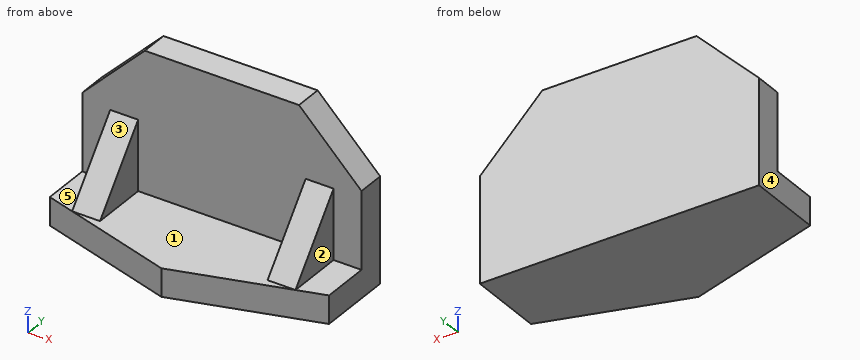
```python
from build123d import *

# Parameters (mm, degrees)
F0_W      = 127
F0_H      = 76.2
F1_DEPTH  = 53.848
F2_W      = 41.148
F2_H      = 63.5
F3_DEPTH  = 127
F5_DEPTH  = 12.7
F7_DEPTH  = 12.7
F8_W      = 12.7
F8_H      = 25.908
F9_DEPTH  = 31.75
F11_DEPTH = 12.7
F13_DEPTH = 12.7


with BuildPart() as f1:
    # F0 (on Front) → F1 (new body)
    with BuildSketch(Plane.XZ):
        with Locations((-17.504597, -0.584449)):
            Rectangle(F0_W, F0_H)
    extrude(amount=F1_DEPTH)

    # F2 (on face) → F3 (cut)
    with BuildSketch(Plane.YZ.offset(45.995403)):
        with Locations((-33.274, 5.765551)):
            Rectangle(F2_W, F2_H)
    extrude(amount=-F3_DEPTH, mode=Mode.SUBTRACT)

    # F4 (on face) → F5 (cut)
    with BuildSketch(Plane.XZ.offset(12.7)):
        Polygon((45.995403, 9.067551), (45.995403, 37.515551), (17.547403, 37.515551), align=None)
        Polygon((-52.556597, 37.515551), (-81.004597, 37.515551), (-81.004597, 9.067551), align=None)
    extrude(amount=-F5_DEPTH, mode=Mode.SUBTRACT)

    # F6 (on face) → F7 (cut)
    with BuildSketch(Plane.XY.offset(-25.984449)):
        Polygon((45.995403, -34.798), (-17.504597, -53.848), (45.995403, -53.848), align=None)
        Polygon((-81.004597, -53.848), (-17.504597, -53.848), (-81.004597, -34.798), align=None)
    extrude(amount=-F7_DEPTH, mode=Mode.SUBTRACT)

    # F8 (on face) → F9 (join)
    with BuildSketch(Plane.XY.offset(-25.984449)):
        with Locations((26.945403, -25.654)):
            Rectangle(F8_W, F8_H)
        with Locations((-61.954597, -25.654)):
            Rectangle(F8_W, F8_H)
    extrude(amount=F9_DEPTH)

    # F10 (on face) → F11 (cut)
    with BuildSketch(Plane.YZ.offset(-55.604597)):
        Polygon((-38.608, -25.984449), (-12.7, 5.765551), (-38.608, 5.765551), align=None)
    extrude(amount=-F11_DEPTH, mode=Mode.SUBTRACT)

    # F12 (on face) → F13 (cut)
    with BuildSketch(Plane.YZ.offset(33.295403)):
        Polygon((-38.608, -25.984449), (-12.7, 5.765551), (-38.608, 5.765551), align=None)
    extrude(amount=-F13_DEPTH, mode=Mode.SUBTRACT)


solid = f1.part
```
The listing builds one solid part. Answer for the finished solid, in the listing's coordinates (mm). Face numbers are marked on the shaded views. A direction names the side the tool comes from. Round coordinates to 2 decimals unless told otherwise and drop trailing zeros. Loops run counter-clockwise (first coordinate to the right, second up) from the corner with the lowest first, then second, coordinate; pieces in that order, holes last.
1) A cutting plane is placed at D-D on y = -7. Determine the outline of the cut face in (x, z), plus the area to 3 significant figures.
Outcome:
outline: (-81, -38.68) - (46, -38.68) - (46, 9.07) - (17.55, 37.52) - (-52.56, 37.52) - (-81, 9.07) - close
area: 8,870 mm2
2) Consider line 1 (X direction, y = -21, z = -15); line 2 (Y direction, x = -28.5, z = -22); line 3 (Z direction, x = -46, y = -14). Determine where each line is inside the solid, lowest interval first.
Outcome:
line 1: x = -68.3 to -55.6, 20.6 to 33.3
line 2: y = -12.7 to 0
line 3: z = -38.68 to -25.98
3) Given P1, Ø14, axis at x = -77, y = -28.5, coming from the +Z side; P2, Ø8, axis at y = -29, z = -8, coming from the -X side; P3, Ø6, axis at x = 8, z = 25, coming from the -Y side; P4, Ø3, axis at x = 18.5, z = -12.5, coming from the +Y side, each flat-ended and moving along its own axis, determine where each tip first touches the part or whether it passes through.
Outcome:
P1: stops at z = -25.98
P2: stops at x = -68.3
P3: stops at y = -12.7
P4: stops at y = 0
4) A cutting plane is placed at A-A on z = -16.5. Determine the outline of the cut face in (x, y).
Outcome:
outline: (-81, -12.7) - (-68.3, -12.7) - (-68.3, -30.87) - (-55.6, -30.87) - (-55.6, -12.7) - (20.6, -12.7) - (20.6, -30.87) - (33.3, -30.87) - (33.3, -12.7) - (46, -12.7) - (46, 0) - (-81, 0) - close
5) A cutting plane is placed at B-B on y = -24. Determine the outline of the cut face in (x, z).
Outcome:
outline: (-81, -38.68) - (46, -38.68) - (46, -25.98) - (33.3, -25.98) - (33.3, -8.08) - (20.6, -8.08) - (20.6, -25.98) - (-55.6, -25.98) - (-55.6, -8.08) - (-68.3, -8.08) - (-68.3, -25.98) - (-81, -25.98) - close
6) For the marked faces 1, 2, 3, 4 and 5, determine the directions among +Z, -Z, +X, -X, +Y, -Y from which every point of the face is accessible in a straight line to the end or side of a thin tool.
Outcome:
face 1: +Z, -Y
face 2: +Z, +X, -Y
face 3: +Z, +X, -X, -Y
face 4: +Z, -Z, -X, +Y, -Y
face 5: +Z, -X, -Y
7) A cutting plane is placed at C-C on x = -50.5. Determine the outline of the cut face in (y, z).
Outcome:
outline: (-43.95, -38.68) - (0, -38.68) - (0, 37.52) - (-12.7, 37.52) - (-12.7, -25.98) - (-43.95, -25.98) - close
